Can you work these out from the model? Positions are in its coordinate system, mm. A direction names the side the tool comes from. Round coordinates to 2 decimals unless told otherwise and drop trailing zeros. Write each loop counter-clockwise with the first axis right and the second up, starting at its lowest first coordinate (ties: lowest second). Pieces come first, ordered by that corner, then holes. Notation, with made-up numbers: M -31,44 L -11,44 A15 cw -11,72 Z; hole C 62,79 d8. An arc over 180 degrees is marked long. Answer as a JSON object with one key per item and string values. Group by question number.
1) I'm going to push flat-ended pins straight in: pin 1 Ø1 at (x, y) = (-24.5, 9) entering from +Z; pin 2 Ø8 at (x, z) = (-24.5, 14) entering from +Y; pin 3 Ø6 at (x, y) = (-14, 11) entering from +Z. Where does each tip first touch, or does it pass through?
2) Please list where these lines run through material, in increasing order: L1, parallel to Z at x = -8, y = 0; L2, parallel to X at y = -2.5, z = 19.5; L3, parallel to Z at x = -13.5, y = -9.5. Write a range as [from, to].
3) Suppose I cut it at B-B, the plane y = -2. Write out the boundary of the cut face in (x, z), and give its area (3 significant figures).
4) Suppose I cut it at A-A, the plane x = -12.5. Write out the boundary of the cut face in (y, z).
5) Suppose I cut it at C-C, the plane z = 18.5. Write out the boundary of the cut face in (x, y), and give its area (3 significant figures).
6) Suppose I cut it at D-D, the plane x = -7.5. Write out the boundary of the cut face in (y, z), and give its area (3 significant figures).
7) On a 3-axis mill with a long thin cutter (end or side, diameter ignored), from which of +Z, -Z, +X, -X, +Y, -Y can I reach the whole of each face in a straight line? I mean faces 1 (the flat face through (-20, 0, 15)), 2 (the flat face through (-10, -6, 15)), 3 (the flat face through (-6, 12, 0)). Say none if no direction works.
from build123d import *

# Parameters (mm, degrees)
SKETCH1_W           = 20
SKETCH1_H           = 12.5
BOSS_EXTRUDE1_DEPTH = 30
SKETCH2_W           = 40
SKETCH2_H           = 40
BOSS_EXTRUDE2_DEPTH = 20
FILLET1_R           = 10


with BuildPart() as part:
    # Sketch1 → Boss-Extrude1 (new body)
    with BuildSketch(Plane.XY):
        with Locations((-20, -6.25)):
            Rectangle(SKETCH1_W, SKETCH1_H)
    extrude(amount=BOSS_EXTRUDE1_DEPTH)

    # Sketch2 → Boss-Extrude2 (add)
    with BuildSketch(Plane.XY):
        with Locations((-10, 7.5)):
            Rectangle(SKETCH2_W, SKETCH2_H)
    extrude(amount=-BOSS_EXTRUDE2_DEPTH)

    # Fillet1
    fillet1_edges = [part.edges().sort_by_distance(p)[0] for p in [
        (10, 27.5, -10),
        (-20, 0, 30),
        (-20, 0, 0),
    ]]
    fillet(fillet1_edges, radius=FILLET1_R)


solid = part.part
Results:
{
 "1": {"pin 1": "z = 0.11", "pin 2": "y = 0", "pin 3": "z = 0.2"},
 "2": {"L1": "[-20, 0]", "L2": "[-30, -10]", "L3": "[-20, 29.99]"},
 "3": {"outline": "M -30,-20 L 10,-20 L 10,0 L -10,0 L -10,26 L -30,26 Z", "area": "1,320 mm^2"},
 "4": {"outline": "M -12.5,-20 L 27.5,-20 L 27.5,0 L 10,0 A10 cw 0,10 L 0,20 A10 ccw -10,30 L -12.5,30 Z"},
 "5": {"outline": "M -30,-12.5 L -10,-12.5 L -10,0 L -30,0 Z", "area": "250 mm^2"},
 "6": {"outline": "M -12.5,-20 L 27.5,-20 L 27.5,0 L -12.5,0 Z", "area": "800 mm^2"},
 "7": {"face 1": "+Z, +X, -X, +Y", "face 2": "+Z, +X, +Y, -Y", "face 3": "+Z, +X, +Y"}
}
